The listing builds one solid part. Answer for the finished solid, in the listing's coordinates (mm). Face numbers are marked on the shaded views. Give positions to 0.01 mm unless a question says otherwise; leave off trailing zeros. Return JSON: item names as keys, results as strings.
from build123d import *

# Parameters (mm, degrees)
UPPER_AIRFRAME_COUPLER_SKETCH_R      = 43.15
UPPER_AIRFRAME_COUPLER_SKETCH_R_2    = 39.975
UPPER_AIRFRAME_COUPLER_EXTRUDE_DEPTH = 25
SHEAR_PIN_BORE_CUT_REACH             = 190.276
SHEAR_PIN_BORE_CUT_END_RADIUS        = 39.975
SHEAR_PIN_BORE_SKETCH_R              = 1.25
SHEAR_PIN_PATTERN_COUNT              = 4


with BuildPart() as part:
    # Ellipsoid Sketch → Ellipsoid Revolve (revolve)
    with BuildSketch(Plane(origin=(0, 0, 0), x_dir=(0, 0, -1), z_dir=(1, 0, 0))):
        with BuildLine():
            Line((-150, 0), (-139.975, 0))
            add(Edge.make_bspline(
                [(0, 39.975), (-139.975, 39.975), (-139.975, 0)],
                knots=[4.71238898, 4.71238898, 4.71238898, 6.283185307, 6.283185307, 6.283185307], degree=2, weights=[1, 0.707106781, 1]))
            Line((0, 39.975), (0, 50))
            add(Edge.make_bspline(
                [(0, 50), (-150, 50), (-150, 0)],
                knots=[4.71238898, 4.71238898, 4.71238898, 6.283185307, 6.283185307, 6.283185307], degree=2, weights=[1, 0.707106781, 1]))
        make_face()
    revolve(axis=Axis((0, 0, -7.5), (0, 0, 1)))

    # Upper Airframe Coupler Sketch → Upper Airframe Coupler Extrude (add)
    with BuildSketch(Plane(origin=(0, 0, 0), x_dir=(-1, 0, 0), z_dir=(0, 0, -1))):
        Circle(UPPER_AIRFRAME_COUPLER_SKETCH_R)
        Circle(UPPER_AIRFRAME_COUPLER_SKETCH_R_2, mode=Mode.SUBTRACT)
    extrude(amount=UPPER_AIRFRAME_COUPLER_EXTRUDE_DEPTH)

    # Upper Airframe Mate Chamfer: read off the stored shape, not the designer's step
    # Upper Airframe Mate Chamfer outline → Upper Airframe Mate Chamfer (revolve, cut)
    with BuildSketch(Plane.XZ):
        Polygon((49.948616721, 6.798616721), (43.15, 0), (50, 0), (50, 6.798616721), align=None)
    revolve(axis=Axis((0, 0, 0), (0, 0, 1)), mode=Mode.SUBTRACT)

    # Shear Pin Bore Cut: up to this cylinder (the profile starts outside it)
    shear_pin_bore_cut_end = Plane(origin=(0, 0, -10), z_dir=(0, 0, -1)) * Cylinder(SHEAR_PIN_BORE_CUT_END_RADIUS, 461.502, mode=Mode.PRIVATE)
    # Shear Pin Bore Sketch → Shear Pin Bore Cut (cut, up to the surface)
    with BuildSketch(Plane(origin=(30.511657608, -30.511657608, 0), x_dir=(-0.7071067811865475, -0.7071067811865477, 0), z_dir=(0.7071067811865477, -0.7071067811865475, 0)), mode=Mode.PRIVATE) as shear_pin_bore_cut_sk1:
        with Locations(Location((0, 10, 0), (0, 0, 180))):
            Circle(SHEAR_PIN_BORE_SKETCH_R)
    shear_pin_bore_cut_tool1 = extrude(shear_pin_bore_cut_sk1.sketch, amount=-SHEAR_PIN_BORE_CUT_REACH, mode=Mode.PRIVATE) - shear_pin_bore_cut_end
    shear_pin_bore_cut = shear_pin_bore_cut_tool1.solids().sort_by_distance((30.511658, -30.511658, -10))[0]
    add(shear_pin_bore_cut, mode=Mode.SUBTRACT)

    # Shear Pin Pattern: Shear Pin Bore Cut ×4 about axis
    shear_pin_pattern_axis = Axis((0, 0, 0), (0, 0, 1))
    for i in range(1, SHEAR_PIN_PATTERN_COUNT):
        add(shear_pin_bore_cut.rotate(shear_pin_pattern_axis, i * 360 / SHEAR_PIN_PATTERN_COUNT), mode=Mode.SUBTRACT)


solid = part.part
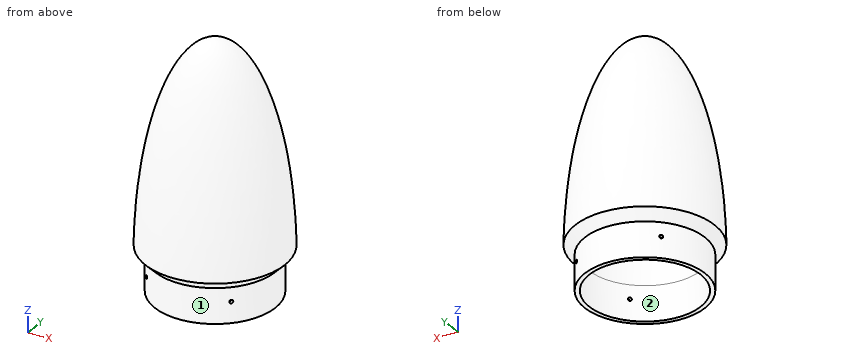
(1) Straight lines are drawn through the part: line 1 along Y through (x, z) = (0, -15.5) (3 decimals); line 2 along Y through (x, z) = (19, 5). For each, find the intervals that lie inside material, in ascending order.
Values follow:
{"line 1": "-43.15 to -39.975, 39.975 to 43.15", "line 2": "-44.24 to -35.14, 35.14 to 44.24"}
(2) Given pin 1 (3 mm diameter, centred on y = -7, z = 97.5, fed in from -X); pin 2 (5 mm diameter, centred on x = -5, y = -6.5, fed in from -Z); pin 3 (5 mm diameter, centred on x = -13, z = 89.5, fed in from -Y), each flat-ended and moving along its own axis, determine where each tip first touches the part or whether it passes through.
Values follow:
{"pin 1": "x = -37.85", "pin 2": "z = 134.87", "pin 3": "y = -38.97"}
(3) Determine the mould class of the marked faces 1 and 2 for opening direction X: released by +X, released by -X, zero draft, split by the parting line, or undercut.
Values follow:
{"face 1": "split by the parting line", "face 2": "undercut"}
